Can you work these out from the model? Positions are in its coordinate system, mm. Round coordinates to 2 decimals unless told otherwise and drop trailing zeros. Write each loop counter-clockwise with the first axis right and the second up, starting at its lowest first coordinate (ties: lowest second). Pieces come first, ordered by that corner, then holes. Notation, with made-up numbers: M -3.5,88.25 L 11.5,88.25 A33 ccw 11.5,126.25 Z; hole C -16,-12.5 d3. An arc over 180 degrees is marked long. Answer as a JSON object with one key per item and string values. Group by question number.
1) I'm going to push flat-ended pins straight in: pin 1 Ø3 at (y, z) = (19, 2) entering from -X; pin 2 Ø4 at (x, z) = (19, 1.5) entering from -Y; pin 3 Ø1.5 at (y, z) = (13.5, 3.5) entering from +X; pin 4 Ø12 at (x, y) = (12, -14.5) entering from -Z. Where does each tip first touch, or does it pass through?
2) If we mould it in two halves opening along Y, with no side actions, what happens to faces 1 (the cylindrical face through (30, 4.57, 4.25)), 2 (the cylindrical face through (-28.27, 11.04, 4.25)), 3 (the cylindrical face through (-19.06, -23.71, 4.25))? For each: +Y half, -Y half, draft (parallel to the pull), parting line (faces both ways), or undercut.
3) Please list where these lines run through material, in increasing order: L1, parallel to Y at x = 0, z = 4.25; L2, parallel to X at y = -21.5, z = 4; L3, parallel to X at y = -11, z = 6.5. Write a range as [from, to].
4) Suppose I cut it at A-A, the plane y = 0. Write out the boundary of the cut face in (x, z), and give its area (3 significant figures).
from build123d import *

# Parameters (mm, degrees)
SKETCH1_R           = 31.75
SKETCH1_R_2         = 12.7
BOSS_EXTRUDE1_DEPTH = 8.382
CUT_EXTRUDE1_DEPTH  = 11.43
CIRPATTERN1_COUNT   = 12


with BuildPart() as part:
    # Sketch1 → Boss-Extrude1 (new body)
    with BuildSketch(Plane.XY):
        Circle(SKETCH1_R)
        Circle(SKETCH1_R_2, mode=Mode.SUBTRACT)
    extrude(amount=BOSS_EXTRUDE1_DEPTH)

    # Sketch2 → Cut-Extrude1 (cut)
    with BuildSketch(Plane.XY.offset(8.382)):
        with BuildLine():
            Line((-7.9375, 30.741805311), (-7.9375, 33.926877276))
            Line((-7.9375, 33.926877276), (7.9375, 33.926877276))
            Line((7.9375, 33.926877276), (7.9375, 30.741805311))
            ThreePointArc((7.9375, 30.741805311), (4.60906835, 30.031219266), (3.176555189, 26.943939587))
            ThreePointArc((3.176555189, 26.943939587), (0, 23.767384397), (-3.176555189, 26.943939587))
            ThreePointArc((-3.176555189, 26.943939587), (-4.60906835, 30.031219266), (-7.9375, 30.741805311))
        make_face()
    cut_extrude1 = extrude(amount=-CUT_EXTRUDE1_DEPTH, mode=Mode.SUBTRACT)

    # CirPattern1: Cut-Extrude1 ×12 about axis
    cirpattern1_axis = Axis((0, 0, 0), (0, 0, 1))
    for i in range(1, CIRPATTERN1_COUNT):
        add(cut_extrude1.rotate(cirpattern1_axis, i * 360 / CIRPATTERN1_COUNT), mode=Mode.SUBTRACT)


solid = part.part
Results:
{
 "1": {"pin 1": "x = -23.75", "pin 2": "y = -23.75", "pin 3": "x = 20.25", "pin 4": "z = 0"},
 "2": {"face 1": "undercut", "face 2": "+Y half", "face 3": "-Y half"},
 "3": {"L1": "[-23.77, -12.7], [12.7, 23.77]", "L2": "[-23.22, -16.07], [-10.88, 10.88], [16.07, 23.22]", "L3": "[-28.37, -25.47], [-21.34, -6.35], [6.35, 21.34], [25.47, 28.37]"},
 "4": {"outline": "M -23.77,0 L -12.7,0 L -12.7,8.38 L -23.77,8.38 Z; M 12.7,0 L 23.77,0 L 23.77,8.38 L 12.7,8.38 Z", "area": "186 mm^2"}
}
